Verification items for the finished model (mm, model axes). Face numbers are marked on the shaded views. A direction names the side the tool comes from. Round coordinates to 2 decimals unless told otherwise and drop trailing zeros. Write each loop counter-clockwise with the first axis right and the second up, starting at its lowest first coordinate (ties: lowest second). Pieces come first, ordered by that corner, then holes. Notation, with made-up numbers: (-11, -4) - (3, -4) arc R19 cw to (3, 10) - close; hole circle Ø7 at (20, 8.5). An arc over 180 degrees is marked (long way). Answer as a JSON object with one key per item and string values.
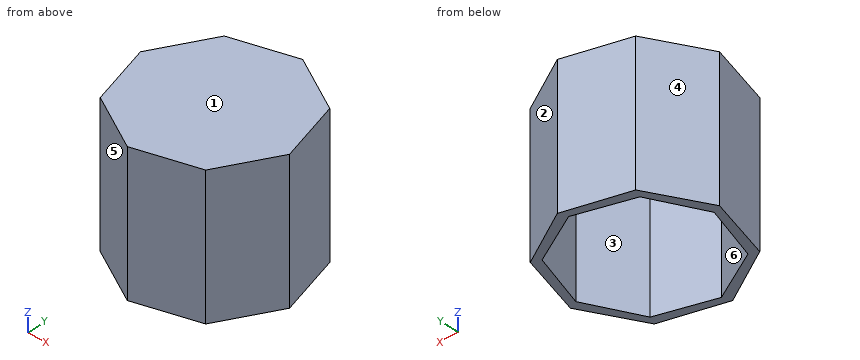
```python
from build123d import *

# Parameters (mm, degrees)
F1_DEPTH = 83.312
F3_DEPTH = 80.772


with BuildPart() as f1:
    # F0 (on Top) → F1 (new body)
    with BuildSketch(Plane.XY):
        Polygon((-31.120799, 39.861828), (-50.192297, 6.180841), (-39.861828, -31.120799), (-6.180841, -50.192297), (31.120799, -39.861828), (50.192297, -6.180841), (39.861828, 31.120799), (6.180841, 50.192297), align=None)
    extrude(amount=F1_DEPTH)

    # F2 (on face) → F3 (cut)
    with BuildSketch(Plane(origin=(0, 0, 0), x_dir=(1, 0, 0), z_dir=(0, 0, -1))):
        Polygon((-4.10583, 45.089582), (-34.786409, 28.979889), (-45.089582, -4.10583), (-28.979889, -34.786409), (4.10583, -45.089582), (34.786409, -28.979889), (45.089582, 4.10583), (28.979889, 34.786409), align=None)
    extrude(amount=-F3_DEPTH, mode=Mode.SUBTRACT)


solid = f1.part
```
Q1. Release check for a two-part mould opening along X. For the marked faces 1, 2, 3 and 4 record: released by +X, released by -X, zero draft, split by the parting line, or undercut.
Geometry check:
{"face 1": "zero draft", "face 2": "released by +X", "face 3": "undercut", "face 4": "released by -X"}
Q2. Gauge pin test, flat ends, axial feed: P1, Ø1.5, axis at y = -10, z = 67, coming from the +X side; P2, Ø12, axis at x = 18, y = -21, coming from the -Z side; P3, Ø2, axis at x = 28, z = 58.5, coming from the +Y side. Record the tip position at first contact, or that the pin passes through.
Geometry check:
{"P1": "stops at x = 48.45", "P2": "stops at z = 80.77", "P3": "stops at y = 38.4"}
Q3. Section check B-B, the plane x = -15. Record the cut outline in (y, z).
Geometry check:
{"outline": "(-45.2, 0) - (-39.37, 0) - (-39.37, 80.77) - (39.14, 80.77) - (39.14, 0) - (44.33, 0) - (44.33, 83.31) - (-45.2, 83.31) - close"}
Q4. Section check A-A, the plane z = 31.5. Record the cut outline in (x, y), then the cut area to 3 significant figures.
Geometry check:
{"outline": "(-50.19, 6.18) - (-39.86, -31.12) - (-6.18, -50.19) - (31.12, -39.86) - (50.19, -6.18) - (39.86, 31.12) - (6.18, 50.19) - (-31.12, 39.86) - close; hole (-45.09, 4.11) - (-34.79, -28.98) - (-4.11, -45.09) - (28.98, -34.79) - (45.09, -4.11) - (34.79, 28.98) - (4.11, 45.09) - (-28.98, 34.79) - close", "area": "1,440 mm2"}
Q5. Set-up check for the marked faces 5 and 6: record each of +Z, -Z, +X, -X, +Y, -Y from which the full face is reachable in a straight line by a thin tool's end or side.
Geometry check:
{"face 5": "+Z, -Z, -X, -Y", "face 6": "-Z"}
Q6. Section check C-C, the plane y = 15.5. Record the cut outline in (x, z).
Geometry check:
{"outline": "(-44.92, 0) - (-39.11, 0) - (-39.11, 80.77) - (38.98, 80.77) - (38.98, 0) - (44.19, 0) - (44.19, 83.31) - (-44.92, 83.31) - close"}
Q7. Material ranges on line 1 along Z through (x, y) = (-2.5, -9.5); line 2 along Y through (x, z) = (23.5, 64); line 3 along X through (y, z) = (24.5, 50.5), recorded low to high. Write a range as [from, to].
Geometry check:
{"line 1": "z = [80.77, 83.31]", "line 2": "y = [-41.97, -36.49], [34.91, 40.39]", "line 3": "x = [-39.82, -34.38], [36.18, 41.7]"}
